Read the model definition and answer for the solid it produces. Units are mm, in the model's axes. Face numbers are marked on the shaded views. A direction names the side the tool comes from. Coordinates: 2 decimals unless noted, no trailing zeros. Order: outer loops, then holes, each group sorted by start corner. A loop starts at its lowest first (then second) coordinate and runs counter-clockwise, first axis right, second up. Notation, with made-up numbers: M -31.75,-38.75 L 0.25,-38.75 A28 cw 0.25,-17.75 Z; hole C 65.5,8.5 d8. An arc over 180 degrees is marked long. Use a Markdown table: item, result. Add a question column.
1) For the marked faces 1 and 2, determine the directions among +Z, -Z, +X, -X, +Y, -Y from which every point of the face is accessible in a straight line to the end or side of a thin tool.
2) Find the intervals of material crossed by probe 1 along Y at (x, z) = (4, 0); probe 2 along Z at (x, y) = (6.75, 0), in increasing order. Write a range as [from, to].
3) Each of these flat-tipped pins is pushed along its axis until it touches: pin 1 Ø4 at (x, y) = (8, 0.5) entering from -Z; pin 2 Ø1.5 at (x, z) = (2.5, -3) entering from +Y. Where does it stop, or does it pass through?
4) Find section B-B on x = 3.5. Write down the section's boundary in (y, z).
5) The mould has two halves that part along Z. Classify the marked faces 3, 4 and 5: released by +Z, released by -Z, zero draft, split by the parting line, or undercut.
6) Find section A-A on x = 5.75. Write down the section's boundary in (y, z).
Autodesk Inventor part; units mm, degrees
ref_plane "YZ Plane" through (0, 0, 0) normal (1, 0, 0) x (0, 1, 0)
ref_plane "XZ Plane" through (0, 0, 0) normal (0, 1, 0) x (-1, 0, 0)
ref_plane "XY Plane" through (0, 0, 0) normal (0, 0, 1) x (1, 0, 0)
sketch "Náčrt1" plane through (0, 0, 0) normal (0, 0, 1) x (1, 0, 0)
  line L0 (0, 0) -> (0, 2.5)
  line L1 (0, 2.5) -> (0.555, 3.4613)
  line L2 (6.6, 3.75) -> (7.85, 5)
  line L3 (7.85, 5) -> (11.6, 5)
  line L4 (11.6, 5) -> (11.6, 4.95)
  arc A0 (11.6, 4.95) -> (13.1, 4.95) centre (12.35, 4.95) ccw
  line L5 (13.1, 4.95) -> (13.1, 6.5)
  line L6 (13.1, 6.5) -> (17.1, 6.5)
  line L7 (17.1, 6.5) -> (17.1, 0)
  line L8 (17.1, 0) -> (0, 0)
  line L9 (1.055, 3.75) -> (0.555, 3.4613)
  line L10 (1.055, 3.75) -> (6.6, 3.75)
  arc A1 (17.1, 2.5) -> (15.1, 6.5) centre (12.1, 2.5) ccw
  dimension "d2" = 30
  dimension "d3" = 45
  dimension "d5" = 6.6
  dimension "d6" = 10
  dimension "d7" = 5
  dimension "d8" = 1.5
  dimension "d9" = 13.1
  dimension "d10" = 17.1
  dimension "d11" = 13
  dimension "d12" = 8.4
  dimension "d32" = 30
  dimension "d34" = 0.5
  dimension "d35" = 7.5
  dimension "d46" = 5
  dimension "d47" = 5
revolve "Rotace1" add sketch "Náčrt1" angle 360 about axis through (17.1, 0, 0) along (-1, 0, 0) contours L0 L1 L9 L10 L2 L3 L4 A0 L5 L6 A1 L7 L8
sketch "Náčrt2" plane through (17.1, 0, 0) normal (1, 0, 0) x (0, 0, -1)
  line L0 (3.1754, 5.5) -> (6.3509, 0)
  line L1 (6.3509, 0) -> (3.1754, -5.5)
  line L2 (3.1754, -5.5) -> (-3.1754, -5.5)
  line L3 (-3.1754, -5.5) -> (-6.3509, 0)
  line L4 (-6.3509, 0) -> (-3.1754, 5.5)
  line L5 (-3.1754, 5.5) -> (3.1754, 5.5)
  circle A0 centre (0, 0) radius 7.7861
  dimension "d14" = 5.5
extrude "Vysunutí1" cut sketch "Náčrt2" against normal through all
sketch "Náčrt4" plane through (0, 0, 0) normal (-1, 0, 0) x (0, 0, 1)
  circle A0 centre (0, 0) radius 3.75
  point P0 (0, 0)
hole "Díra1" at (0, 0, 0) direction (1, 0, 0) diameter 6 end through all
thread "Závit1"
move or copy body "Posunout těleso1" bodies to move or copy 1 copy no rotation origin (0, 0, 0) rotation axis (0, 0, 1) rotation angle 180 translate (13.1, 0, 0)
properties part number "Cap03" material "ČSN 12 050 (1.1201, C45)"
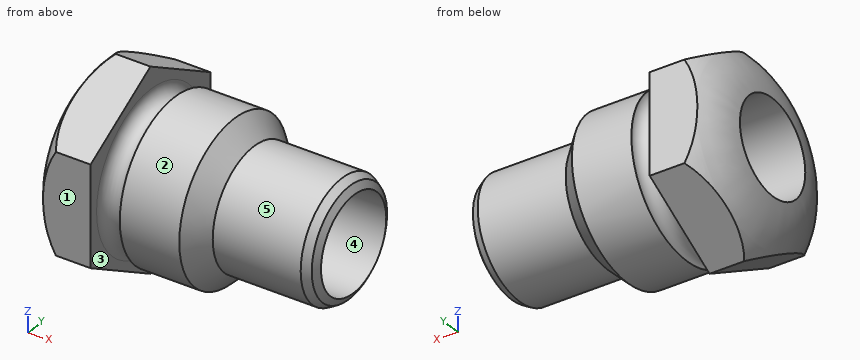
Check result:
| question | item | result |
|---|---|---|
| 1 | face 1 | +Z, -Z, +X, -X, -Y |
| 1 | face 2 | +X |
| 2 | probe 1 | y = [-5, -3], [3, 5] |
| 2 | probe 2 | z = [-3.75, -3], [3, 3.75] |
| 3 | pin 1 | stops at z = -4.23 |
| 3 | pin 2 | stops at y = 4.47 |
| 4 | outline | C 0,0 d10; hole C 0,0 d6 |
| 5 | face 3 | zero draft |
| 5 | face 4 | undercut |
| 5 | face 5 | split by the parting line |
| 6 | outline | C 0,0 d9; hole C 0,0 d6 |
